Part model, mm, in its own coordinate system. Face numbers are marked on the shaded views. A direction names the side the tool comes from. Coordinates: 2 decimals unless noted, no trailing zeros. Loops run counter-clockwise (first coordinate to the right, second up) from the corner with the lowest first, then second, coordinate; pieces in that order, holes last. Notation, with made-up numbers: (-7.75, 66.5) - (41.25, 66.5) arc R13 ccw to (41.25, 76.5) - close; hole circle Ø3 at (34.25, 3.5). An arc over 180 degrees is marked (long way). Answer as CSV lines item,"result".
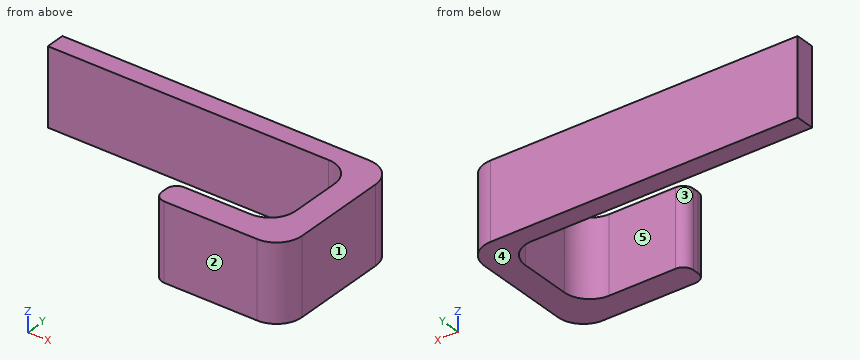
from build123d import *

# Parameters (mm, degrees)
F1_DEPTH = 19.05


with BuildPart() as f1:
    # F0 (on Top) → F1 (new body)
    with BuildSketch(Plane.XY):
        with BuildLine():
            Line((76.453999, 0), (0, 0))
            Line((0, 0), (0, -4.7625))
            Line((0, -4.7625), (69.85, -4.7625))
            ThreePointArc((69.85, -4.7625), (74.340128, -6.622372), (76.2, -11.1125))
            Line((76.2, -11.1125), (76.2, -23.8125))
            ThreePointArc((76.2, -23.8125), (74.340128, -28.302628), (69.85, -30.1625))
            Line((69.85, -30.1625), (53.34, -30.1625))
            ThreePointArc((53.34, -30.1625), (51.543949, -30.906449), (50.8, -32.7025))
            Line((50.8, -32.7025), (50.8, -34.226499))
            ThreePointArc((50.8, -34.226499), (51.543949, -36.022551), (53.34, -36.766499))
            Line((53.34, -36.766499), (76.453999, -36.766499))
            ThreePointArc((76.453999, -36.766499), (80.944127, -34.906627), (82.803999, -30.416499))
            Line((82.803999, -30.416499), (82.803999, -6.35))
            ThreePointArc((82.803999, -6.35), (80.944127, -1.859872), (76.453999, 0))
        make_face()
    extrude(amount=F1_DEPTH)


solid = f1.part
Q1. Two-plate mould, pull along Y, no slides. Class the marked faces 1, 2 and 3: released by +Y, released by -Y, zero draft, split by the parting line, or undercut.
Results:
face 1,"zero draft"
face 2,"released by -Y"
face 3,"undercut"
Q2. Saw through at B-B (z = 2.25). Give the cut face in (x, y), then the cut area to 3 significant figures.
Results:
outline,"(0, -4.76) - (69.85, -4.76) arc R6.35 cw to (76.2, -11.11) - (76.2, -23.81) arc R6.35 cw to (69.85, -30.16) - (53.34, -30.16) arc R2.54 ccw to (50.8, -32.7) - (50.8, -34.23) arc R2.54 ccw to (53.34, -36.77) - (76.45, -36.77) arc R6.35 ccw to (82.8, -30.42) - (82.8, -6.35) arc R6.35 ccw to (76.45, 0) - (0, 0) - close"
area,"771 mm^2"
Q3. Which spindle directions (+Z, -Z, +X, -X, +Y, -Y) get a long thin tool onto all of the face, cutting with end or side? Do the marked faces 4 and 5. Say none if no direction does.
Results:
face 4,"-Z, +X, -X, +Y, -Y"
face 5,"+Z, -Z, -X"
Q4. Flat gauge pins, fed straight in: pin 1 (1.2 mm diameter, centred on y = -33.5, z = 13.5, fed in from -X); pin 2 (2 mm diameter, centred on x = 21, z = 6, fed in from -Y); pin 3 (1 mm diameter, centred on y = -28, z = 6, fed in from -X). Where does each tip first touch, or does it go through?
Results:
pin 1,"stops at x = 50.8"
pin 2,"stops at y = -4.76"
pin 3,"stops at x = 74.13"
Q5. Saw through at D-D (x = 26.5). Give the cut face in (y, z).
Results:
outline,"(-4.76, 0) - (0, 0) - (0, 19.05) - (-4.76, 19.05) - close"
Q6. Saw through at C-C (y = -21). Give the cut face in (x, z), then the cut area to 3 significant figures.
Results:
outline,"(76.2, 0) - (82.8, 0) - (82.8, 19.05) - (76.2, 19.05) - close"
area,"126 mm^2"
Q7. Saw through at A-A (x = 58.5). Give the cut face in (y, z).
Results:
outline,"(-36.77, 0) - (-30.16, 0) - (-30.16, 19.05) - (-36.77, 19.05) - close; (-4.76, 0) - (0, 0) - (0, 19.05) - (-4.76, 19.05) - close"
Q8. Wall check: L1, parallel to Y at x = 58.5, z = 11.5; L2, parallel to Y at x = 20.5, z = 5; L3, parallel to X at y = -18.5, z = 11. Give the ranges that are in metal, low to high.
Results:
L1,"y = -36.77 to -30.16, -4.76 to 0"
L2,"y = -4.76 to 0"
L3,"x = 76.2 to 82.8"
